```python
from build123d import *

# Parameters (mm, degrees)
F0_R     = 10
F0_R_2   = 7.5
F0_W     = 11.8
F0_H     = 17.1
F1_DEPTH = 1.5


# Not quite as in the source:
# - ends of sketch curves that miss each other by under 0.0002 mm in the source are joined


with BuildPart() as f1:
    # F0 (on Top) → F1 (new body, symmetric)
    with BuildSketch(Plane.XY):
        Polygon((-46.9999983907, 3.8743e-06), (-46.9999983907, -4.9999961257), (-43.9999983907, -4.9999961257), (-43.9999983907, -14.9999961257), (-46.9999983907, -14.9999961257), (-46.9999983907, -24.9999961257), (-43.9999983907, -24.9999961257), (-43.9999983907, -34.9999961257), (-46.9999983907, -34.9999961257), (-46.9999983907, -44.9999961257), (-43.9999983907, -44.9999961257), (-43.9999983907, -54.9999961257), (-46.9999983907, -54.9999961257), (-46.9999983907, -64.9999961257), (-43.9999983907, -64.9999961257), (-43.9999983907, -74.9999961257), (-46.9999983907, -74.9999961257), (-46.9999983907, -89.9999961257), (-31.9999983907, -89.9999961257), (-31.9999983907, -86.9999961257), (-21.9999983907, -86.9999961257), (-21.9999983907, -89.9999961257), (-11.9999983907, -89.9999961257), (-11.9999983907, -86.9999961257), (-1.9999983907, -86.9999961257), (-1.9999983907, -89.9999961257), (8.0000016093, -89.9999961257), (8.0000016093, -86.9999961257), (18.0000016093, -86.9999961257), (18.0000016093, -89.9999961257), (28.0000016093, -89.9999961257), (28.0000016093, -86.9999961257), (38.0000016093, -86.9999961257), (38.0000016093, -89.9999961257), (53.0000016093, -89.9999961257), (53.0000030994, -75.968132019), (50.0000030994, -75.968132019), (50.0000030994, -65.968132019), (53.0000030994, -65.968132019), (53.0000030994, -55.968132019), (50.0000030994, -55.968132019), (50.0000030994, -45.968132019), (53.0000030994, -45.968132019), (53.0000030994, -35.968132019), (50.0000030994, -35.968132019), (50.0000030994, -25.968132019), (53.0000030994, -25.968132019), (53.0000030994, -15.968132019), (50.0000030994, -15.968132019), (50.0000030994, -5.968132019), (53.0000030994, -5.968132019), (53.0000030994, 3.8743e-06), (53.0000030994, 4.031867981), (50.0000030994, 4.031867981), (50.0000030994, 14.031867981), (53.0000030994, 14.031867981), (53.0000030994, 24.031867981), (50.0000030994, 24.031867981), (50.0000030994, 34.031867981), (53.0000030994, 34.031867981), (53.0000030994, 44.031867981), (50.0000030994, 44.031867981), (50.0000030994, 54.031867981), (53.0000030994, 54.031867981), (53.0000030994, 64.031867981), (50.0000030994, 64.031867981), (50.0000030994, 74.031867981), (53.0000030994, 74.031867981), (53.0000030994, 90.0000038743), (38.0000016093, 90.0000035763), (38.0000016093, 87.0000035763), (28.0000016093, 87.0000035763), (28.0000016093, 90.0000035763), (18.0000016093, 90.0000035763), (18.0000016093, 87.0000035763), (8.0000016093, 87.0000035763), (8.0000016093, 90.0000035763), (-1.9999983907, 90.0000035763), (-1.9999983907, 87.0000035763), (-11.9999983907, 87.0000035763), (-11.9999983907, 90.0000035763), (-21.9999983907, 90.0000035763), (-21.9999983907, 87.0000035763), (-31.9999983907, 87.0000035763), (-31.9999983907, 90.0000035763), (-46.9999983907, 90.0000035763), (-46.9999983907, 75.0000038743), (-43.9999983907, 75.0000038743), (-43.9999983907, 65.0000038743), (-46.9999983907, 65.0000038743), (-46.9999983907, 55.0000038743), (-43.9999983907, 55.0000038743), (-43.9999983907, 45.0000038743), (-46.9999983907, 45.0000038743), (-46.9999983907, 35.0000038743), (-43.9999983907, 35.0000038743), (-43.9999983907, 25.0000038743), (-46.9999983907, 25.0000038743), (-46.9999983907, 15.0000038743), (-43.9999983907, 15.0000038743), (-43.9999983907, 5.0000038743), (-46.9999983907, 5.0000038743), align=None)
        with Locations((-10.3999983907, 3.8743e-06)):
            Circle(F0_R, mode=Mode.SUBTRACT)
        with Locations((33.0000030994, -69.9999961257)):
            Circle(F0_R_2, mode=Mode.SUBTRACT)
        with Locations((-26.9999983907, 70.0000035763)):
            Circle(F0_R_2, mode=Mode.SUBTRACT)
        with Locations((32.1000030994, 3.8743e-06)):
            Rectangle(F0_W, F0_H, mode=Mode.SUBTRACT)
    extrude(amount=F1_DEPTH, both=True)


solid = f1.part
```
Here's how the part is built. I have some questions about the finished solid (model axes, mm). Give positions to 0.01 mm unless a question says otherwise; leave off trailing zeros. Loops run counter-clockwise (first coordinate to the right, second up) from the corner with the lowest first, then second, coordinate; pieces in that order, holes last. Notation, with made-up numbers: (36, 37.5) -> (90, 37.5) arc R8 cw to (90, 43.5) -> close; hole circle Ø4 at (54, -12). An arc over 180 degrees is marked (long way). Use one line per item in the form item = value. Start each with the question number.
1) Imagine slicing it at A-A (x = -25.5). Please give me the cut outline in (y, z), then the cut area to 3 significant figures.
2) Thinking about a two-plate mould opening in Y: for faces 1 (the face through (2, 1, -1.5)), 2 (the face through (-0.86, 3, -0.02)), 3 (the face through (-27.976, 77.436, -0.021)), which applies, +Y half, -Y half, draft (parallel to the pull), parting line (faces both ways), or undercut?
3) Imagine slicing it at B-B (z = 0.95). Count the separate pieces of the cut face and the enclosed holes in it, then the cut area to 3 significant figures.
4) Please list where these lines run through material, in increasing order: line 1 along Y through (x, z) = (10, -0.6); line 2 along X through (y, z) = (75.5, -0.55); line 3 along Y through (x, z) = (-4, -0.1).
5) Imagine slicing it at C-C (x = -5.5). Please give me the cut outline in (y, z).
6) Imagine slicing it at D-D (x = 13). Please give me the cut outline in (y, z), then the cut area to 3 significant figures.
7) For P1, Ø1, axis at x = -8.5, z = 0.5, coming from the +Y side, with a flat end and sliding along its axis, tell me the tip position at first contact or that it passes through.
Check values:
q1.outline = (-87, -1.5) -> (62.65, -1.5) -> (62.65, 1.5) -> (-87, 1.5) -> close; (77.35, -1.5) -> (87, -1.5) -> (87, 1.5) -> (77.35, 1.5) -> close
q1.area = 478 mm^2
q2.face_1 = draft
q2.face_2 = undercut
q2.face_3 = undercut
q3.separate_pieces = 1
q3.enclosed_holes = 4
q3.area = 16,400 mm^2
q4.line_1 = -87 to 87
q4.line_2 = -47 to -32.1, -21.9 to 53
q4.line_3 = -87 to -7.68, 7.68 to 87
q5.outline = (-87, -1.5) -> (-8.72, -1.5) -> (-8.72, 1.5) -> (-87, 1.5) -> close; (8.72, -1.5) -> (87, -1.5) -> (87, 1.5) -> (8.72, 1.5) -> close
q6.outline = (-87, -1.5) -> (87, -1.5) -> (87, 1.5) -> (-87, 1.5) -> close
q6.area = 522 mm^2
q7.P1 = 87
